Check sheet for the modelled part. Datum: model origin and axes. Units: mm. A direction names the side the tool comes from. Round coordinates to 2 decimals unless told otherwise and drop trailing zeros. Order: outer loops, then holes, each group sorted by start corner. A loop starts at its lowest first (then second) coordinate and runs counter-clockwise, first axis right, second up. Notation, with made-up numbers: M -33,7 L 12,7 A19 cw 12,39 Z; hole C 89.5,56.25 d4. An arc over 180 degrees is marked long. One line per item, written item: value. Start each with the question number.
(1) Cross-section at A-A, the plane x = -33.5. Enter the section's corners in (y, z), and give its area (3 significant figures).
(2) Depth check by flat-ended pin: pin 1 Ø8 at (y, z) = (-11, 11.5) entering from -X; pin 2 Ø1.5 at (x, z) = (-4, 2.5) entering from -Y; pin 3 Ø1 at (y, z) = (-10, 2.5) entering from -X. Enter the tip coordinate at first touch or a pass-through.
(3) Access from +Z, -Z, +X, -X, +Y, -Y to the whole of each face (thin tool, end or side, straight path). Record for faces 1 (the face through (-10, 6.75, 10)), 2 (the face through (6.11, -5.32, 18.5)), 3 (the face through (56, -7, 5)), 4 (the face through (6.11, 5.32, 18.5)).
(4) Release check for a two-part mould opening along Z. For faces 5 (the face through (56, 7, 5)), 6 (the face through (-48.675, -0.094, 16.958)), 7 (the face through (55.86, 11.974, 8.352)) record: released by +Z, released by -Z, zero draft, split by the parting line, or undercut.
(5) Thickness scan on L1, parallel to Z at x = 54, y = 10.25; L2, parallel to Y at x = -55, z = 14.5; L3, parallel to X at y = 8.25, z = 16.75. Record the ranges inside material, lowest first.
(6) Cross-section at C-C, the plane x = 30.5. Enter the section's corners in (y, z).
(7) Cross-section at B-B, the plane x = 50.5. Enter the section's corners in (y, z), and give its area (3 significant figures).
from build123d import *

# Parameters (mm, degrees)
ESQUISSE1_W                  = 132
ESQUISSE1_H                  = 30
BOSS_EXTRU_1_DEPTH           = 20
ESQUISSE3_W                  = 112
ESQUISSE3_H                  = 8.25
ENL_V_MAT_EXTRU_1_DEPTH      = 71.576199954
ENL_V_MAT_EXTRU_2_REACH      = 74.312
ESQUISSE4_R                  = 1.375
ESQUISSE5_R                  = 2
ENL_V_MAT_EXTRU_3_DEPTH      = 80
CONG_1_R                     = 5
CONG_2_R                     = 5
CONG_3_R                     = 1
ENL_V_MAT_EXTRU_4_DEPTH      = 7
ENL_V_MAT_EXTRU_4_DEPTH_BACK = 7
CONG_4_R                     = 2
ENL_V_MAT_EXTRU_5_DEPTH      = 71.576200076
ENL_V_MAT_EXTRU_5_DEPTH_BACK = 71.576200076


with BuildPart() as part:
    # Esquisse1 → Boss.-Extru.1 (new body)
    with BuildSketch(Plane.XY):
        Rectangle(ESQUISSE1_W, ESQUISSE1_H)
    extrude(amount=BOSS_EXTRU_1_DEPTH)

    # Esquisse3 → Enlèv. mat.-Extru.1 (cut, through all)
    with BuildSketch(Plane.XY.offset(20)):
        with Locations((-10, 10.875)):
            Rectangle(ESQUISSE3_W, ESQUISSE3_H)
        with Locations((-10, -10.875)):
            Rectangle(ESQUISSE3_W, ESQUISSE3_H)
    extrude(amount=-ENL_V_MAT_EXTRU_1_DEPTH, mode=Mode.SUBTRACT)

    # Esquisse4 → Enlèv. mat.-Extru.2 (cut, up to next)
    with BuildSketch(Plane.XZ.offset(6.75), mode=Mode.PRIVATE) as enl_v_mat_extru_2_sk1:
        with Locations(Location((-61, 7, 0), (0, 0, 270))):
            Circle(ESQUISSE4_R)
    enl_v_mat_extru_2_tool1 = extrude(enl_v_mat_extru_2_sk1.sketch, amount=-ENL_V_MAT_EXTRU_2_REACH, mode=Mode.PRIVATE) & part.part
    add(enl_v_mat_extru_2_tool1.solids().sort_by_distance((-61, -6.75, 7))[0], mode=Mode.SUBTRACT)

    # Esquisse5 → Enlèv. mat.-Extru.3 (cut)
    with BuildSketch(Plane.ZY.offset(-46)):
        with Locations(Location((7, -10.5, 0), (0, 0, 270))):
            Circle(ESQUISSE5_R)
        with Locations(Location((7, 10.5, 0), (0, 0, 270))):
            Circle(ESQUISSE5_R)
    extrude(amount=-ENL_V_MAT_EXTRU_3_DEPTH, mode=Mode.SUBTRACT)

    # Congé1
    cong_1_edges = [part.edges().sort_by_distance(p)[0] for p in [
        (56, -15, 0),
        (56, -15, 20),
        (56, 15, 0),
        (56, 15, 20),
    ]]
    fillet(cong_1_edges, radius=CONG_1_R)

    # Congé2
    cong_2_edges = [part.edges().sort_by_distance(p)[0] for p in [
        (-10, 6.75, 0),
        (-10, 6.75, 20),
        (-10, -6.75, 0),
        (-10, -6.75, 20),
    ]]
    fillet(cong_2_edges, radius=CONG_2_R)

    # Congé3
    # the kernel refuses this fillet: 1 mm, written as the material it adds along each edge
    with BuildSketch(Plane(origin=(46, -6.75, 15), x_dir=(0, -1, 0), z_dir=(0, 0, -1))) as cong_3_piece_1:
        with BuildLine():
            CenterArc((CONG_3_R, CONG_3_R), CONG_3_R, 180, 90)
            Line((0, CONG_3_R), (0, 0))
            Line((0, 0), (CONG_3_R, 0))
        make_face()
    extrude(amount=10)
    with BuildSketch(Plane(origin=(46, 6.75, 15), x_dir=(0, 1, 0), z_dir=(0, 0, -1))) as cong_3_piece_2:
        with BuildLine():
            CenterArc((CONG_3_R, -CONG_3_R), CONG_3_R, 90, 90)
            Line((0, -CONG_3_R), (0, 0))
            Line((0, 0), (CONG_3_R, 0))
        make_face()
    extrude(amount=10)
    with BuildSketch(Plane(origin=(46, -1.75, 15), x_dir=(0, 0.7515057138603058, 0.6597265812708415), z_dir=(0, 0.6597265812708415, -0.7515057138603058))) as cong_3_piece_3_section:
        with BuildLine():
            CenterArc((5 + CONG_3_R, -CONG_3_R), CONG_3_R, 90, 90)
            Line((5, -CONG_3_R), (5, 0))
            Line((5, 0), (5 + CONG_3_R, 0))
        make_face()
    cong_3_piece_3 = revolve(axis=Axis((46, -1.75, 15), (1, 0, 0)), revolution_arc=138.720976341, mode=Mode.PRIVATE)
    cong_3_piece_3 = split(cong_3_piece_3, bisect_by=Plane(origin=(46, -1.75, 20), z_dir=(0, 0, -1)), keep=Keep.TOP, mode=Mode.PRIVATE)
    add(cong_3_piece_3)
    with BuildSketch(Plane(origin=(46, 1.75, 15), x_dir=(0, -0.7515057138603058, 0.6597265812708415), z_dir=(0, -0.6597265812708415, -0.7515057138603058))) as cong_3_piece_4_section:
        with BuildLine():
            CenterArc((5 + CONG_3_R, CONG_3_R), CONG_3_R, 180, 90)
            Line((5, CONG_3_R), (5, 0))
            Line((5, 0), (5 + CONG_3_R, 0))
        make_face()
    cong_3_piece_4 = revolve(axis=Axis((46, 1.75, 15), (-1, 0, 0)), revolution_arc=138.720976341, mode=Mode.PRIVATE)
    cong_3_piece_4 = split(cong_3_piece_4, bisect_by=Plane(origin=(46, 1.75, 20), z_dir=(0, 0, -1)), keep=Keep.TOP, mode=Mode.PRIVATE)
    add(cong_3_piece_4)
    with BuildSketch(Plane(origin=(46, 1.75, 5), x_dir=(0, -0.7515057138603056, -0.6597265812708417), z_dir=(0, -0.6597265812708417, 0.7515057138603056))) as cong_3_piece_5_section:
        with BuildLine():
            CenterArc((5 + CONG_3_R, -CONG_3_R), CONG_3_R, 90, 90)
            Line((5, -CONG_3_R), (5, 0))
            Line((5, 0), (5 + CONG_3_R, 0))
        make_face()
    cong_3_piece_5 = revolve(axis=Axis((46, 1.75, 5), (1, 0, 0)), revolution_arc=138.720976341, mode=Mode.PRIVATE)
    cong_3_piece_5 = split(cong_3_piece_5, bisect_by=Plane(origin=(46, 1.75, 0), z_dir=(0, 0, 1)), keep=Keep.TOP, mode=Mode.PRIVATE)
    add(cong_3_piece_5)
    with BuildSketch(Plane(origin=(46, -1.75, 5), x_dir=(0, 0.7515057138603056, -0.6597265812708416), z_dir=(0, 0.6597265812708416, 0.7515057138603056))) as cong_3_piece_6_section:
        with BuildLine():
            CenterArc((5 + CONG_3_R, CONG_3_R), CONG_3_R, 180, 90)
            Line((5, CONG_3_R), (5, 0))
            Line((5, 0), (5 + CONG_3_R, 0))
        make_face()
    cong_3_piece_6 = revolve(axis=Axis((46, -1.75, 5), (-1, 0, 0)), revolution_arc=138.720976341, mode=Mode.PRIVATE)
    cong_3_piece_6 = split(cong_3_piece_6, bisect_by=Plane(origin=(46, -1.75, 0), z_dir=(0, 0, 1)), keep=Keep.TOP, mode=Mode.PRIVATE)
    add(cong_3_piece_6)

    # Esquisse7 → Enlèv. mat.-Extru.4 (cut, two sides: drawn at the far end of the back side and taken through both)
    with BuildSketch(Plane(origin=(0, 0, 0), x_dir=(1, 0, 0), z_dir=(0, 1, 0)).offset(-ENL_V_MAT_EXTRU_4_DEPTH_BACK)):
        Polygon((66, -12), (9.544438686, 0), (66, 0), align=None)
    extrude(amount=ENL_V_MAT_EXTRU_4_DEPTH + ENL_V_MAT_EXTRU_4_DEPTH_BACK, mode=Mode.SUBTRACT)

    # Congé4
    cong_4_edges = [part.edges().sort_by_distance(p)[0] for p in [
        (-66, -6.75, 10),
        (-66, 0, 20),
        (-66, 6.75, 10),
        (-66, 0, 0),
        (-66, -5.285533906, 1.464466094),
        (-66, 5.285533906, 1.464466094),
        (-66, 5.285533906, 18.535533906),
        (-66, -5.285533906, 18.535533906),
    ]]
    fillet(cong_4_edges, radius=CONG_4_R)

    # Esquisse8 → Enlèv. mat.-Extru.5 (cut, two sides: drawn at the far end of the back side and taken through both)
    with BuildSketch(Plane(origin=(0, 0, 0), x_dir=(1, 0, 0), z_dir=(0, 1, 0)).offset(-ENL_V_MAT_EXTRU_5_DEPTH_BACK)):
        Polygon((-36, -20), (-66, -20), (-66, -14), (-61, -14), align=None)
    extrude(amount=ENL_V_MAT_EXTRU_5_DEPTH + ENL_V_MAT_EXTRU_5_DEPTH_BACK, mode=Mode.SUBTRACT)


solid = part.part
Values found:
1. outline: M -6.75,5 A5 ccw -1.75,0 L 1.75,0 A5 ccw 6.75,5 L 6.75,15 A5 ccw 1.75,20 L -1.75,20 A5 ccw -6.75,15 Z
1. area: 249 mm^2
2. pin 1: x = 45.66
2. pin 2: y = -6.43
2. pin 3: x = 46
3. face 1: +Z, -Z, -X, +Y
3. face 2: +Z, -X, -Y
3. face 3: -Z, +X
3. face 4: +Z, -X, +Y
4. face 5: zero draft
4. face 6: released by +Z
4. face 7: undercut
5. L1: 0.01 to 5.02, 8.98 to 19.99
5. L2: -6.75 to 6.75
5. L3: 46 to 66
6. outline: M -6.75,5 A5 ccw -6.72,4.45 L 6.72,4.45 A5 ccw 6.75,5 L 6.75,15 A5 ccw 1.75,20 L -1.75,20 A5 ccw -6.75,15 Z
7. outline: M -15,5 A5 ccw -10,0 L -7,0 L -7,8.71 L 7,8.71 L 7,0 L 10,0 A5 ccw 15,5 L 15,15 A5 ccw 10,20 L -10,20 A5 ccw -15,15 Z; hole C -10.5,7 d4; hole C 10.5,7 d4
7. area: 432 mm^2
